For this review, take the finished solid that the model builds, in its own axes (mm). Round coordinates to 2 decimals unless told otherwise and drop trailing zeros. Order: outer loops, then holes, each group sorted by start corner. A loop starts at its lowest first (then second) coordinate and runs counter-clockwise, first axis right, second up.
```python
from build123d import *

# Parameters (mm, degrees)
ESBO_O1_W                = 58
ESBO_O1_H                = 2.5
RESSALTO_EXTRUS_O1_DEPTH = 107.92
FILETE1_R                = 5.5
ESBO_O2_R                = 9
CORTE_EXTRUS_O1_DEPTH    = 111.42
ESBO_O5_R                = 11.5
CORTE_EXTRUS_O2_DEPTH    = 111.42


with BuildPart() as part:
    # Esboço1 → Ressalto-extrusão1 (new body)
    with BuildSketch(Plane(origin=(0, 0, 0), x_dir=(1, 0, 0), z_dir=(0, 1, 0))):
        with Locations((22.039718439, -2.022727273)):
            Rectangle(ESBO_O1_W, ESBO_O1_H)
    extrude(amount=RESSALTO_EXTRUS_O1_DEPTH)

    # Filete1
    filete1_edges = [part.edges().sort_by_distance(p)[0] for p in [
        (51.039718439, 107.92, 2.022727273),
        (-6.960281561, 107.92, 2.022727273),
        (51.039718439, 0, 2.022727273),
        (-6.960281561, 0, 2.022727273),
    ]]
    fillet(filete1_edges, radius=FILETE1_R)

    # Esboço2 → Corte-extrusão1 (cut)
    with BuildSketch(Plane.XY.offset(3.272727273)):
        with Locations((22.039718439, 79.92)):
            Circle(ESBO_O2_R)
        with Locations((22.039718439, 45.4387)):
            Circle(ESBO_O2_R)
    extrude(amount=-CORTE_EXTRUS_O1_DEPTH, mode=Mode.SUBTRACT)

    # Esboço5 → Corte-extrusão2 (cut)
    with BuildSketch(Plane.XY.offset(3.272727273)):
        with Locations((22.039718439, 21.2424)):
            Circle(ESBO_O5_R)
    extrude(amount=-CORTE_EXTRUS_O2_DEPTH, mode=Mode.SUBTRACT)


solid = part.part
```
Q1. Take a section at B-B, the plane y = 79.92. State the section outline as (x, z) points, plus the area to 3 significant figures.
Q2. Mouldability with a two-part tool opening along X and no side actions: class faces 1 (the face through (-5.39, 1.65, 2.01)), 2 (the face through (15, 53, 0.773)), 3 (the face through (49.47, 1.65, 2.01)), 4 (the face through (19.547, 10.016, 2.04)) as +X half, -X half, draft (parallel to the pull), parting line (faces both ways), or undercut.
Q3. Wall thickness on line 1 (X direction, y = 45.5, z = 2.55); line 2 (Y direction, x = 22.5, z = 2.65); line 3 (Y direction, x = 46, z = 2.05): over which ranges is each line inside the solid? List them lowest first.
Q4. Take a section at D-D, the plane x = 17. State the section outline as (y, z) points.
Q5. Take a section at C-C, the plane z = 2.85. State the section outline as (x, y) points.
Q6. Take a section at A-A, the plane x = 25.5. State the section outline as (y, z) points, plus the area to 3 significant figures.
Working result:
1. outline: (-6.96, 0.77) - (13.04, 0.77) - (13.04, 3.27) - (-6.96, 3.27) - close; (31.04, 0.77) - (51.04, 0.77) - (51.04, 3.27) - (31.04, 3.27) - close
1. area: 100 mm2
2. face 1: -X half
2. face 2: draft
2. face 3: +X half
2. face 4: undercut
3. line 1: x = -6.96 to 13.04, 31.04 to 51.04
3. line 2: y = 0 to 9.75, 32.73 to 36.45, 54.43 to 70.93, 88.91 to 107.92
3. line 3: y = 0.02 to 107.9
4. outline: (0, 0.77) - (10.91, 0.77) - (10.91, 3.27) - (0, 3.27) - close; (31.58, 0.77) - (37.98, 0.77) - (37.98, 3.27) - (31.58, 3.27) - close; (52.9, 0.77) - (72.46, 0.77) - (72.46, 3.27) - (52.9, 3.27) - close; (87.38, 0.77) - (107.92, 0.77) - (107.92, 3.27) - (87.38, 3.27) - close
5. outline: (-6.96, 5.5) arc R5.5 ccw to (-1.46, 0) - (45.54, 0) arc R5.5 ccw to (51.04, 5.5) - (51.04, 102.42) arc R5.5 ccw to (45.54, 107.92) - (-1.46, 107.92) arc R5.5 ccw to (-6.96, 102.42) - close; hole circle Ø23 at (22.04, 21.24); hole circle Ø18 at (22.04, 45.44); hole circle Ø18 at (22.04, 79.92)
6. outline: (0, 0.77) - (10.28, 0.77) - (10.28, 3.27) - (0, 3.27) - close; (32.21, 0.77) - (37.13, 0.77) - (37.13, 3.27) - (32.21, 3.27) - close; (53.75, 0.77) - (71.61, 0.77) - (71.61, 3.27) - (53.75, 3.27) - close; (88.23, 0.77) - (107.92, 0.77) - (107.92, 3.27) - (88.23, 3.27) - close
6. area: 132 mm2
